from build123d import *

# Parameters (mm, degrees)
BOSS_EXTRUDE1_DEPTH = 5
SKETCH2_W           = 99
SKETCH2_H           = 10
BOSS_EXTRUDE2_DEPTH = 10
BOSS_EXTRUDE3_DEPTH = 10
SKETCH4_R           = 1.75
CUT_EXTRUDE1_DEPTH  = 100


with BuildPart() as part:
    # Sketch1 → Boss-Extrude1 (new body)
    with BuildSketch(Plane.XY):
        Polygon((67.175144213, 60.104076401), (60.104076401, 67.175144213), (93.338122667, 100.409190479), (100.409190479, 93.338122667), align=None)
    extrude(amount=-BOSS_EXTRUDE1_DEPTH)

    # Sketch2 → Boss-Extrude2 (add)
    with BuildSketch(Plane(origin=(96.873656573, 96.873656573, 0), x_dir=(0, 0, -1), z_dir=(0.707106781, 0.707106781, 0))):
        with Locations((49.5, 0)):
            Rectangle(SKETCH2_W, SKETCH2_H)
    extrude(amount=BOSS_EXTRUDE2_DEPTH)

    # Sketch3 → Boss-Extrude3 (add)
    with BuildSketch(Plane(origin=(3.535533906, -3.535533906, 0), x_dir=(0, 0, -1), z_dir=(0.707106781, -0.707106781, 0))):
        Polygon((5, 100), (22.25340152, 137.000038963), (5, 137.000038963), align=None)
    extrude(amount=-BOSS_EXTRUDE3_DEPTH)

    # Sketch4 → Cut-Extrude1 (cut, through all)
    with BuildSketch(Plane.XY):
        with Locations((67.175144213, 67.175144213)):
            Circle(SKETCH4_R)
    extrude(amount=-CUT_EXTRUDE1_DEPTH, mode=Mode.SUBTRACT)


solid = part.part
The listing builds one solid part. Answer for the finished solid, in the listing's coordinates (mm). A direction names the side the tool comes from. Coordinates: 2 decimals unless noted, no trailing zeros. Order: outer loops, then holes, each group sorted by start corner. A loop starts at its lowest first (then second) coordinate and runs counter-clockwise, first axis right, second up. Notation, with made-up numbers: (1, 33) -> (26, 33) arc R12 cw to (26, 45) -> close; hole circle Ø8 at (56.5, 25). An arc over 180 degrees is marked (long way). Answer in a Markdown table with one row per item. Add a question column.
Item 1: Find section B-B (x = 97.5). Write down the section's boundary in (y, z).
Item 2: Find section C-C (y = 81). Write down the section's boundary in (x, z).
Item 3: Each of these flat-tipped pins is pushed along its axis until it touches: P1, Ø12, axis at x = 72.5, y = 66.5, coming from the -Z side; P2, Ø1, axis at x = 73.5, y = 67, coming from the -Z side; P3, Ø4, axis at y = 100.5, z = -10.5, coming from the -X side. Where does it stop, or does it pass through?
Item 4: Find section A-A (z = -74.5). Write down the section's boundary in (x, y), then the cut area to 4 significant figures.
Item 5: Find the intervals of material crossed by L1, parallel to Y at x = 105.5, z = -58; L2, parallel to X at y = 103.5, z = -36; L3, parallel to Y at x = 102.5, z = -73, in increasing order. Write a range as from..to.
Item 6: Which of the six approach directions +Z, -Z, +X, -X, +Y, -Y give full straight-line access (tool end or side, diameter ignored) to faces 1 (the face through (84, 83, 0)), 2 (the face through (96.824, 96.923, -60.089))?
Result set:
| question | item | result |
|---|---|---|
| 1 | outline | (90.43, -20.33) -> (96.25, -22.25) -> (96.25, -99) -> (104.57, -99) -> (104.57, 0) -> (90.43, 0) -> close |
| 2 | outline | (73.93, -9.45) -> (88.07, -14.12) -> (88.07, 0) -> (73.93, 0) -> close |
| 3 | P1 | stops at z = -7 |
| 3 | P2 | stops at z = -5 |
| 3 | P3 | stops at x = 91.43 |
| 4 | outline | (93.34, 100.41) -> (100.41, 93.34) -> (107.48, 100.41) -> (100.41, 107.48) -> close |
| 4 | area | 100.0 mm² |
| 5 | L1 | y = 98.43..102.39 |
| 5 | L2 | x = 96.43..104.39 |
| 5 | L3 | y = 95.43..105.39 |
| 6 | face 1 | +Z, +X, -X, +Y, -Y |
| 6 | face 2 | -Z, -X, -Y |
